Read the model definition and answer for the solid it produces. Units are mm, in the model's axes. Face numbers are marked on the shaded views. A direction names the side the tool comes from. Coordinates: 2 decimals unless noted, no trailing zeros. Loops run counter-clockwise (first coordinate to the right, second up) from the corner with the lowest first, then second, coordinate; pieces in that order, holes last.
Autodesk Inventor part; units mm, degrees
ref_plane "YZ Plane" through (0, 0, 0) normal (1, 0, 0) x (0, 1, 0)
ref_plane "XZ Plane" through (0, 0, 0) normal (0, 1, 0) x (-1, 0, 0)
ref_plane "XY Plane" through (0, 0, 0) normal (0, 0, 1) x (1, 0, 0)
sketch "Sketch1" plane through (0, 0, 0) normal (0, 0, 1) x (1, 0, 0)
  line L0 (-23.95, -23.95) -> (23.95, -23.95)
  line L1 (23.95, -23.95) -> (23.95, 23.95)
  line L2 (23.95, 23.95) -> (-23.95, 23.95)
  line L3 (-23.95, 23.95) -> (-23.95, -23.95)
  line L4 (-23.95, -23.95) -> (23.95, 23.95) construction
  line L5 (23.95, -23.95) -> (-23.95, 23.95) construction
  line L6 (28.95, 28.95) -> (28.95, -28.95)
  line L7 (28.95, -28.95) -> (-28.95, -28.95)
  line L8 (-28.95, -28.95) -> (-28.95, 28.95)
  line L9 (-28.95, 28.95) -> (28.95, 28.95)
  point P0 (0, 0)
  dimension "d0" = 47.9
  dimension "d1" = 47.9
  dimension "d2" = 5
extrude "Extrusion1" add sketch "Sketch1" along normal blind 85
sketch "Sketch2" plane through (0, 0, 85) normal (0, 0, 1) x (1, 0, 0)
  line L0 (-23.95, 23.95) -> (23.95, 23.95)
  line L1 (-23.95, -23.95) -> (23.95, -23.95)
  line L2 (23.95, -23.95) -> (23.95, 23.95)
  line L3 (23.95, 23.95) -> (-23.95, 23.95)
  line L4 (-23.95, 23.95) -> (-23.95, -23.95)
  line L5 (-23.95, -23.95) -> (23.95, 23.95) construction
  line L6 (23.95, -23.95) -> (-23.95, 23.95) construction
  point P0 (0, 0)
extrude "Extrusion2" add sketch "Sketch2" against normal blind 5
sketch "Sketch3" plane through (0, 0, 85) normal (0, 0, 1) x (1, 0, 0)
  circle A0 centre (0, 0) radius 16
  dimension "d7" = 32
extrude "Extrusion3" cut sketch "Sketch3" along normal blind 8
sketch "Sketch4" plane through (-28.95, -28.95, 0) normal (-1, 0, 0) x (0, 0, 1)
  point P0 (0, 28.95)
sketch "Sketch5" plane through (0, 0, 80) normal (0, 0, -1) x (-1, 0, 0)
  line L0 (23.95, 23.95) -> (-23.95, 23.95)
  line L1 (-23.95, 23.95) -> (23.95, 23.95)
  line L2 (23.95, 23.95) -> (23.95, -23.9872)
  line L3 (23.95, -23.9872) -> (-23.95, -23.9872)
  line L4 (-23.95, -23.9872) -> (-23.95, 23.95)
  point P0 (0, 0)
extrude "Extrusion4" add sketch "Sketch5" along normal blind 10
sketch "Sketch6" plane through (0, 0, 70) normal (0, 0, -1) x (-1, 0, 0)
  point P0 (0, 0)
sketch "Sketch7" plane through (0, 0, 70) normal (0, 0, -1) x (-1, 0, 0)
  circle A0 centre (0, 0) radius 16
  dimension "d12" = 32
extrude "Extrusion5" cut sketch "Sketch7" against normal blind 10
sketch "Sketch8" plane through (0, 0, 85) normal (0, 0, 1) x (1, 0, 0)
  circle A0 centre (0, 0) radius 13
  dimension "d15" = 26
extrude "Extrusion6" cut sketch "Sketch8" against normal blind 5
properties part number "banebot soporte"
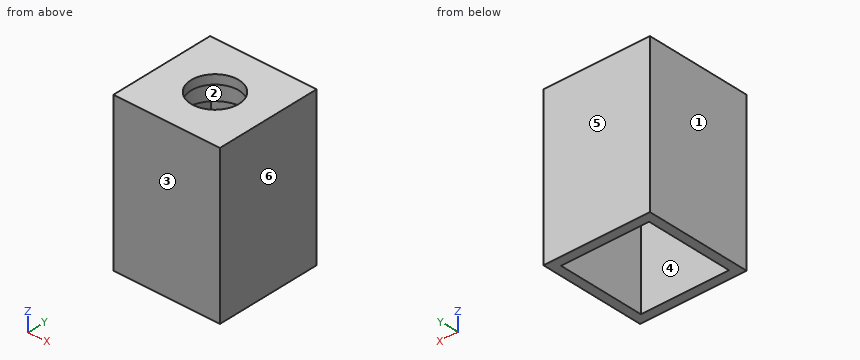
Q1. Straight lines are drawn through the part: probe 1 along Y at (x, z) = (-8, 32.5); probe 2 along Y at (x, z) = (0, 81.1). For each, find the intervals that lie inside material, in ascending order.
Findings below:
probe 1: y = -28.95 to -23.95, 23.95 to 28.95
probe 2: y = -28.95 to -13, 13 to 28.95
Q2. A cutting plane is placed at D-D (y = -21). Give the vertices of the cut face in (x, z), then the cut area to 3 significant figures.
Findings below:
outline: (-28.95, 0) - (-23.95, 0) - (-23.95, 70) - (23.95, 70) - (23.95, 0) - (28.95, 0) - (28.95, 85) - (-28.95, 85) - close
area: 1,570 mm2
Q3. Flat-ended cylindrical pins translate along their axes: pin 1 Ø24 at (x, y) = (-1.5, 11.5) entering from -Z; pin 2 Ø16 at (x, y) = (2.5, -5.5) entering from -Z; pin 3 Ø19 at (x, y) = (0, 0) entering from -Z. Find the tip coordinate at first contact, or state that the pin passes through.
Findings below:
pin 1: stops at z = 70
pin 2: stops at z = 80
pin 3: passes through
Q4. Which of the six approach directions +Z, -Z, +X, -X, +Y, -Y give full straight-line access (tool end or side, diameter ignored) to the marked faces 1 and 2?
Findings below:
face 1: +Z, -Z, -X, +Y, -Y
face 2: -Z
Q5. A cutting plane is placed at A-A (y = 0). Give the vertices of the cut face in (x, z), then the cut area to 3 significant figures.
Findings below:
outline: (-28.95, 0) - (-23.95, 0) - (-23.95, 70) - (-16, 70) - (-16, 80) - (-13, 80) - (-13, 85) - (-28.95, 85) - close; (13, 80) - (16, 80) - (16, 70) - (23.95, 70) - (23.95, 0) - (28.95, 0) - (28.95, 85) - (13, 85) - close
area: 1,120 mm2
Q6. A cutting plane is placed at B-B (z = 55). Give the vertices of the cut face in (x, y), then the cut area to 3 significant figures.
Findings below:
outline: (-28.95, -28.95) - (28.95, -28.95) - (28.95, 28.95) - (-28.95, 28.95) - close; hole (-23.95, -23.95) - (23.95, -23.95) - (23.95, 23.95) - (-23.95, 23.95) - close
area: 1,060 mm2
Q7. Determine the mould class of the marked faces 3, 4, 5 and 6 for opening direction Y: +Y half, -Y half, draft (parallel to the pull), parting line (faces both ways), or undercut.
Findings below:
face 3: -Y half
face 4: undercut
face 5: +Y half
face 6: draft
